```python
from build123d import *

# Parameters (mm, degrees)
F0_W     = 254.508
F0_H     = 43.18
F0_W_2   = 12.7
F0_H_2   = 3.048
F1_DEPTH = 3.175


# Not quite as in the source:
# - a feature names something its author has since deleted; it is built from what else it names


with BuildPart() as f1:
    # F0 (on Top) → F1 (new body)
    with BuildSketch(Plane.XY):
        with Locations((0.254, 0.1834339905)):
            Rectangle(F0_W, F0_H)
        with Locations((-95.25, -17.2155660095)):
            Rectangle(F0_W_2, F0_H_2, mode=Mode.SUBTRACT)
        with Locations((-6.35, -17.2155660095)):
            Rectangle(F0_W_2, F0_H_2, mode=Mode.SUBTRACT)
        with Locations((88.9, -17.2155660095)):
            Rectangle(F0_W_2, F0_H_2, mode=Mode.SUBTRACT)
        with Locations((-95.25, 17.8364339905)):
            Rectangle(F0_W_2, F0_H_2, mode=Mode.SUBTRACT)
        with Locations((-6.35, 17.8364339905)):
            Rectangle(F0_W_2, F0_H_2, mode=Mode.SUBTRACT)
        Polygon((78.9593234658, -3.1185660095), (76.4378011227, -3.1185660095), (76.4378011227, 4.5014339905), (78.9593234658, 4.5014339905), (111.8867844343, 4.5014339905), (111.8867844343, -3.1185660095), align=None, mode=Mode.SUBTRACT)
        with Locations((88.9, 17.8364339905)):
            Rectangle(F0_W_2, F0_H_2, mode=Mode.SUBTRACT)
    extrude(amount=F1_DEPTH)


solid = f1.part
```
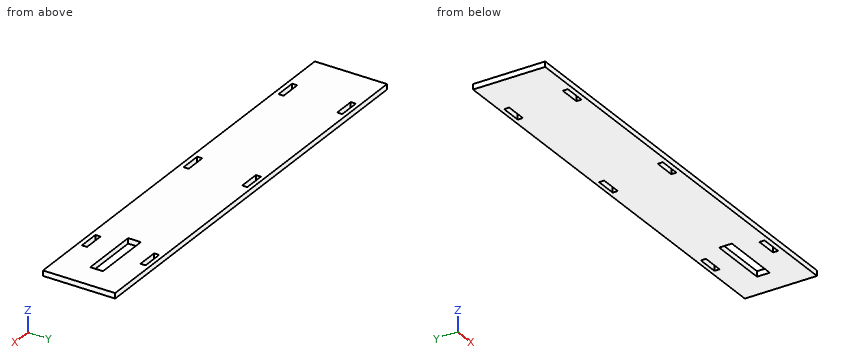
Geometry: final body of the model. Coordinates: model frame, mm. Round coordinates to 2 decimals unless told otherwise and drop trailing zeros. Order: outer loops, then holes, each group sorted by start corner. A loop starts at its lowest first (then second) coordinate and runs counter-clockwise, first axis right, second up. Notation, with made-up numbers: M 29.5,7 L 36.5,7 A20 cw 36.5,12 Z; hole C -10.75,62.25 d2. An arc over 180 degrees is marked long. Use one line per item in the form item = value. Start each with the question number.
Q1. Material intervals for line 1 (X direction, y = 17, z = 1.9); line 2 (Y direction, x = -97.5, z = 1); line 3 (Y direction, x = 89.5, z = 0.6), sorted ascending. Write a range as [from, to].
Q2. Cut plane B-B (y = 0.5). Return loops of the section in (x, z) (3 decimals), and give its area (3 significant figures).
Q3. Cut plane A-A (x = 104.5). Return loops of the section in (y, z) (3 decimals), and give its area (3 significant figures).
Q4. Cut plane C-C (z = 2.35). Count the separate pieces of the cut face and the enclosed holes in it, and give its area (3 significant figures).
Geometry results:
q1.line_1 = [-127, -101.6], [-88.9, -12.7], [0, 82.55], [95.25, 127.51]
q1.line_2 = [-21.41, -18.74], [-15.69, 16.31], [19.36, 21.77]
q1.line_3 = [-21.41, -18.74], [-15.69, -3.12], [4.5, 16.31], [19.36, 21.77]
q2.outline = M -127,0 L 76.438,0 L 76.438,3.175 L -127,3.175 Z; M 111.887,0 L 127.508,0 L 127.508,3.175 L 111.887,3.175 Z
q2.area = 696 mm^2
q3.outline = M -21.407,0 L -3.119,0 L -3.119,3.175 L -21.407,3.175 Z; M 4.501,0 L 21.773,0 L 21.773,3.175 L 4.501,3.175 Z
q3.area = 113 mm^2
q4.separate_pieces = 1
q4.enclosed_holes = 7
q4.area = 10,500 mm^2
